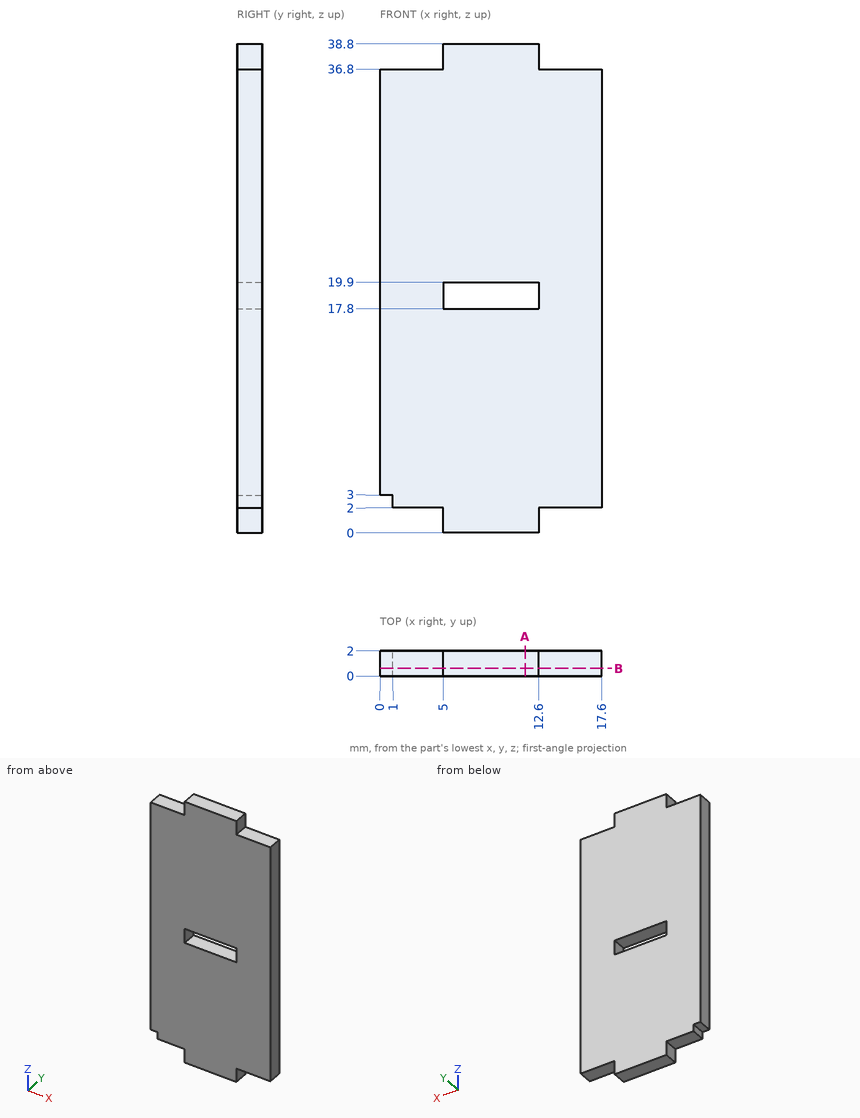
Answer from the drawing. Dimensions are ordinates in mm from the lowest x, y and z of the part. Round coordinates to 2 decimals unless told otherwise and drop trailing zeros. Order: outer loops, then holes, each group sorted by start corner. A loop starts at its lowest first (then second) coordinate and runs counter-clockwise, first axis right, second up. Notation, with made-up numbers: (74.5, 75) - (105.5, 75) arc R20 cw to (105.5, 91) - close; hole circle Ø4 at (-32.75, -13.75). An arc over 180 degrees is marked (long way). Put each result on its own line as item: value. Start each with the question number.
(1) Straight lines are drawn through the part: probe 1 along Z at (x, y) = (12.25, 0.9); probe 2 along Z at (x, y) = (2, 1.2). For each, find the intervals that lie inside material, in ascending order. Write a range as from..to.
(2) Given P1, Ø0.6, axis at y = 1.5, z = 38, coming from the +X side; P2, Ø1, axis at x = 15.5, y = 0.5, coming from the +Z side; P3, Ø0.5, axis at x = 0.5, y = 1, coming from the -Z side, each flat-ended and moving along its own axis, determine where each tip first touches the part or whether it passes through.
(3) Find section B-B (y = 0.6). Give the vertices of the cut face in (x, z), plus the area to 3 significant figures.
(4) Find section A-A (x = 11.5). Give the vertices of the cut face in (y, z), plus the area to 3 significant figures.
Reply:
1. probe 1: 0..17.8, 19.9..38.8
1. probe 2: 2..36.8
2. P1: x = 12.6
2. P2: z = 36.8
2. P3: z = 3
3. outline: (0, 3) - (1, 3) - (1, 2) - (5, 2) - (5, 0) - (12.6, 0) - (12.6, 2) - (17.6, 2) - (17.6, 36.8) - (12.6, 36.8) - (12.6, 38.8) - (5, 38.8) - (5, 36.8) - (0, 36.8) - close; hole (5, 17.8) - (12.6, 17.8) - (12.6, 19.9) - (5, 19.9) - close
3. area: 626 mm^2
4. outline: (0, 0) - (2, 0) - (2, 17.8) - (0, 17.8) - close; (0, 19.9) - (2, 19.9) - (2, 38.8) - (0, 38.8) - close
4. area: 73.4 mm^2
